Read the model definition and answer for the solid it produces. Units are mm, in the model's axes. Face numbers are marked on the shaded views. Coordinates: 2 decimals unless noted, no trailing zeros. Write each loop counter-clockwise with the first axis right and the second up, starting at its lowest first coordinate (ties: lowest second). Pieces come first, ordered by that corner, then holes.
(1) Section B-B on z = 25.5 is taken. State how many separate pieces and enclosed holes the cut face has, then the cut area to 3 significant figures.
(2) The mould has two halves that part along Y. Classify the marked faces 1, 2 and 3: +Y half, -Y half, draft (parallel to the pull), parting line (faces both ways), or undercut.
(3) Section A-A on y = 117.5 is taken. Write down the section's boundary in (x, z), then the cut area to 3 significant figures.
(4) Given pin 1 (12 mm diameter, centred on x = -11.5, y = 141, fed in from -Z); pin 2 (2 mm diameter, centred on x = 40.5, z = 52.5, fed in from +Y), each flat-ended and moving along its own axis, determine where each tip first touches the part or whether it passes through.
(5) Find the intervals of material crossed by probe 1 along Y at (x, z) = (43.5, 15); probe 2 along Y at (x, z) = (27.5, -88); probe 3 along Y at (x, z) = (-22.5, -20), in increasing order.
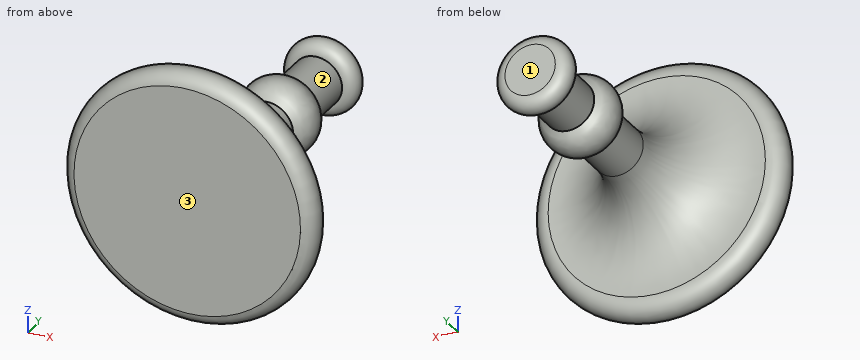
from build123d import *


with BuildPart() as part:
    # Sketch1 → Revolve1 (revolve)
    with BuildSketch(Plane.XY, mode=Mode.PRIVATE) as revolve1_sk:
        with BuildLine():
            Line((0, 0), (0, 220))
            Line((0, 220), (20, 220))
            ThreePointArc((20, 220), (30, 210), (20, 200))
            Line((20, 200), (20, 160))
            ThreePointArc((20, 160), (30.908939581, 142.185606368), (20, 124.371212737))
            Line((20, 124.371212737), (20, 84.371212737))
            ThreePointArc((20, 84.371212737), (39.870136229, 39.766347153), (86.319801124, 24.704973424))
            ThreePointArc((86.319801124, 24.704973424), (100, 14.116257913), (90, 0))
            Line((90, 0), (0, 0))
        make_face()
    revolve(revolve1_sk.sketch.rotate(Axis((0, 0, 0), (0, 1, 0)), 90), axis=Axis((0, 0, 0), (0, 1, 0)))


solid = part.part
Response:
1. separate pieces: 3
1. enclosed holes: 0
1. area: 7,870 mm2
2. face 1: +Y half
2. face 2: undercut
2. face 3: -Y half
3. outline: circle Ø40 at (0, 0)
3. area: 1,260 mm2
4. pin 1: stops at z = -30.4
4. pin 2: stops at y = 26.2
5. probe 1: y = 0 to 34.93
5. probe 2: y = 0.64 to 23.91
5. probe 3: y = 0 to 51.05, 136.57 to 147.8
